The listing builds one solid part. Answer for the finished solid, in the listing's coordinates (mm). Face numbers are marked on the shaded views. A direction names the side the tool comes from. Coordinates: 2 decimals unless noted, no trailing zeros. Write each loop counter-clockwise with the first axis right and the second up, starting at its lowest first coordinate (ties: lowest second). Pieces come first, ordered by that corner, then holes.
(1) Which of the six approach directions +Z, -Z, +X, -X, +Y, -Y give full straight-line access (tool end or side, diameter ignored) to the marked faces 5, 6, 7 and 8?
(2) Straight lines are drawn through the part: line 1 (X direction, y = 89.4, z = 17.65); line 2 (Y direction, x = 0, z = 11.75); line 3 (Z direction, x = 12, y = 24). For each, find the intervals that lie inside material, in ascending order.
(3) The part is cut by section C-C on y = 30. Determine the outline of the cut face in (x, z), plus the area to 3 significant figures.
(4) The part is cut by section D-D on y = 13. Determine the outline of the cut face in (x, z).
(5) Given P1, Ø6, axis at x = 15.5, y = 37, coming from the -Z side; P2, Ø10, axis at y = 102.5, z = 6.5, coming from the +X side; P3, Ø4, axis at x = -10.5, y = 89.4, coming from the +Z side, each flat-ended and moving along its own axis, determine where each tip first touches the part or whether it passes through.
(6) The part is cut by section B-B on y = 103.9. Determine the outline of the cut face in (x, z).
(7) For a pull along X with two mould halves and no side action, classify the marked faces 1, 2, 3 and 4 as +X half, -X half, draft (parallel to the pull), parting line (faces both ways), or undercut.
(8) The part is cut by section A-A on z = 0. Determine the outline of the cut face in (x, y), plus the area to 3 significant figures.
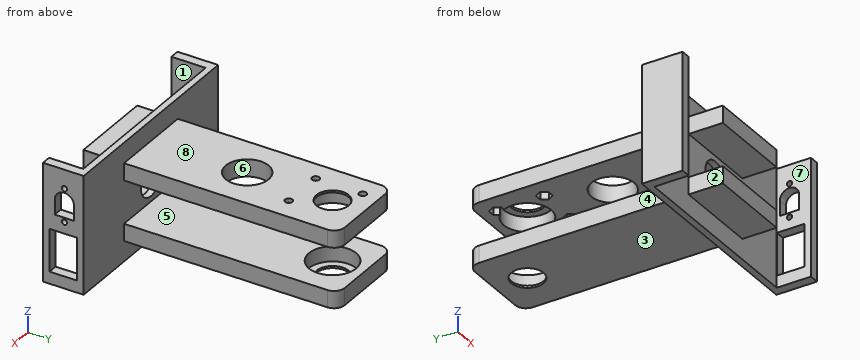
from build123d import *

# Parameters (mm, degrees)
SKETCH1_W            = 100
SKETCH1_H            = 55
BOSS_EXTRUDE1_DEPTH  = 19
SKETCH2_W            = 91
SKETCH2_H            = 91
CUT_EXTRUDE1_DEPTH   = 16
CUT_EXTRUDE3_REACH   = 102
SKETCH3_R            = 1.25
CUT_EXTRUDE13_REACH  = 102
SKETCH15_W           = 19.8
SKETCH15_H           = 12.9
BOSS_EXTRUDE2_START  = -19
SKETCH6_W            = 40
SKETCH6_H            = 8
BOSS_EXTRUDE2_DEPTH  = 119
SKETCH7_R            = 11.05
CUT_EXTRUDE5_DEPTH   = 7
SKETCH8_R            = 7.55
CUT_EXTRUDE6_DEPTH   = 1
FILLET1_R            = 5
FILLET1_OF_MIRROR2_R = 5
CUT_EXTRUDE7_REACH   = 21
SKETCH9_R            = 7.5
CUT_EXTRUDE10_REACH  = 47.5
SKETCH12_R           = 10
CUT_EXTRUDE11_REACH  = 47.5
SKETCH13_R           = 1.75
CUT_EXTRUDE12_DEPTH  = 6


with BuildPart() as part:
    # Sketch1 → Boss-Extrude1 (new body)
    with BuildSketch(Plane(origin=(0, 0, 0), x_dir=(1, 0, 0), z_dir=(0, 1, 0))):
        Rectangle(SKETCH1_W, SKETCH1_H)
    extrude(amount=BOSS_EXTRUDE1_DEPTH)

    # Sketch2 → Cut-Extrude1 (cut)
    with BuildSketch(Plane.XZ):
        Rectangle(SKETCH2_W, SKETCH2_H)
    extrude(amount=-CUT_EXTRUDE1_DEPTH, mode=Mode.SUBTRACT)

    # Sketch3 → Cut-Extrude3 (cut, up to next)
    with BuildSketch(Plane(origin=(50, 0, 0), x_dir=(0, 0, -1), z_dir=(1, 0, 0)), mode=Mode.PRIVATE) as cut_extrude3_sk1:
        with Locations((-18.75, 10)):
            Circle(SKETCH3_R)
    cut_extrude3_tool1 = extrude(cut_extrude3_sk1.sketch, amount=-CUT_EXTRUDE3_REACH, mode=Mode.PRIVATE) & part.part
    add(cut_extrude3_tool1.solids().sort_by_distance((50, 10, 18.75))[0], mode=Mode.SUBTRACT)
    # Sketch3 → Cut-Extrude3 (cut, up to next)
    with BuildSketch(Plane(origin=(50, 0, 0), x_dir=(0, 0, -1), z_dir=(1, 0, 0)), mode=Mode.PRIVATE) as cut_extrude3_sk2:
        with Locations((-3.25, 10)):
            Circle(SKETCH3_R)
    cut_extrude3_tool2 = extrude(cut_extrude3_sk2.sketch, amount=-CUT_EXTRUDE3_REACH, mode=Mode.PRIVATE) & part.part
    add(cut_extrude3_tool2.solids().sort_by_distance((50, 10, 3.25))[0], mode=Mode.SUBTRACT)
    # Sketch3 → Cut-Extrude3 (cut, up to next)
    with BuildSketch(Plane(origin=(50, 0, 0), x_dir=(0, 0, -1), z_dir=(1, 0, 0)), mode=Mode.PRIVATE) as cut_extrude3_sk3:
        with BuildLine():
            Line((-5.272727273, 5.5), (-5.272727273, 14.5))
            Line((-5.272727273, 14.5), (-12.278409091, 14.5))
            ThreePointArc((-12.278409091, 14.5), (-16.778409091, 10), (-12.278409091, 5.5))
            Line((-12.278409091, 5.5), (-5.272727273, 5.5))
        make_face()
    cut_extrude3_tool3 = extrude(cut_extrude3_sk3.sketch, amount=-CUT_EXTRUDE3_REACH, mode=Mode.PRIVATE) & part.part
    add(cut_extrude3_tool3.solids().sort_by_distance((50, 10, 10.590569))[0], mode=Mode.SUBTRACT)

    # Sketch15 → Cut-Extrude13 (cut, up to next)
    with BuildSketch(Plane(origin=(50, 0, 0), x_dir=(0, 0, -1), z_dir=(1, 0, 0)), mode=Mode.PRIVATE) as cut_extrude13_sk1:
        with Locations((12, 9.5)):
            Rectangle(SKETCH15_W, SKETCH15_H)
    cut_extrude13_tool1 = extrude(cut_extrude13_sk1.sketch, amount=-CUT_EXTRUDE13_REACH, mode=Mode.PRIVATE) & part.part
    add(cut_extrude13_tool1.solids().sort_by_distance((50, 9.5, -12))[0], mode=Mode.SUBTRACT)

    # Sketch6 → Boss-Extrude2 (add)
    with BuildSketch(Plane(origin=(0, 19, 0), x_dir=(1, 0, 0), z_dir=(0, 1, 0)).offset(BOSS_EXTRUDE2_START)):
        with Locations((0, -14)):
            Rectangle(SKETCH6_W, SKETCH6_H)
    boss_extrude2 = extrude(amount=BOSS_EXTRUDE2_DEPTH)

    # Sketch7 → Cut-Extrude5 (cut)
    with BuildSketch(Plane(origin=(0, 0, 10), x_dir=(-1, 0, 0), z_dir=(0, 0, -1))):
        with Locations((0, 103.9)):
            Circle(SKETCH7_R)
    cut_extrude5 = extrude(amount=-CUT_EXTRUDE5_DEPTH, mode=Mode.SUBTRACT)

    # Sketch8 → Cut-Extrude6 (cut)
    with BuildSketch(Plane.XY.offset(18)):
        with Locations((0, 103.9)):
            Circle(SKETCH8_R)
    cut_extrude6 = extrude(amount=-CUT_EXTRUDE6_DEPTH, mode=Mode.SUBTRACT)

    # Fillet1
    fillet1_edges = [part.edges().sort_by_distance(p)[0] for p in [
        (-20, 119, 14),
        (20, 119, 14),
    ]]
    fillet(fillet1_edges, radius=FILLET1_R)

    # Mirror2: Boss-Extrude2, Cut-Extrude5, Cut-Extrude6 across plane
    add(boss_extrude2.mirror(Plane.XY))
    add(cut_extrude5.mirror(Plane.XY), mode=Mode.SUBTRACT)
    add(cut_extrude6.mirror(Plane.XY), mode=Mode.SUBTRACT)

    # Fillet1 of Mirror2
    fillet1_of_mirror2_edges = [part.edges().sort_by_distance(p)[0] for p in [
        (-20, 119, -14),
        (20, 119, -14),
    ]]
    fillet(fillet1_of_mirror2_edges, radius=FILLET1_OF_MIRROR2_R)

    # Sketch9 → Cut-Extrude7 (cut, up to next)
    with BuildSketch(Plane(origin=(0, 19, 0), x_dir=(1, 0, 0), z_dir=(0, 1, 0)), mode=Mode.PRIVATE) as cut_extrude7_sk1:
        Circle(SKETCH9_R)
    cut_extrude7_tool1 = extrude(cut_extrude7_sk1.sketch, amount=-CUT_EXTRUDE7_REACH, mode=Mode.PRIVATE) & part.part
    add(cut_extrude7_tool1.solids().sort_by_distance((0, 19, 0))[0], mode=Mode.SUBTRACT)

    # Sketch12 → Cut-Extrude10 (cut, up to next)
    with BuildSketch(Plane.XY.offset(18), mode=Mode.PRIVATE) as cut_extrude10_sk1:
        with Locations((0, 64)):
            Circle(SKETCH12_R)
    cut_extrude10_tool1 = extrude(cut_extrude10_sk1.sketch, amount=-CUT_EXTRUDE10_REACH, mode=Mode.PRIVATE) & part.part
    add(cut_extrude10_tool1.solids().sort_by_distance((0, 64, 18))[0], mode=Mode.SUBTRACT)

    # Sketch13 → Cut-Extrude11 (cut, up to next)
    with BuildSketch(Plane.XY.offset(18), mode=Mode.PRIVATE) as cut_extrude11_sk1:
        with Locations((-10.5, 89.4)):
            Circle(SKETCH13_R)
    cut_extrude11_tool1 = extrude(cut_extrude11_sk1.sketch, amount=-CUT_EXTRUDE11_REACH, mode=Mode.PRIVATE) & part.part
    add(cut_extrude11_tool1.solids().sort_by_distance((-10.5, 89.4, 18))[0], mode=Mode.SUBTRACT)
    # Sketch13 → Cut-Extrude11 (cut, up to next)
    with BuildSketch(Plane.XY.offset(18), mode=Mode.PRIVATE) as cut_extrude11_sk2:
        with Locations((-10.5, 111.4)):
            Circle(SKETCH13_R)
    cut_extrude11_tool2 = extrude(cut_extrude11_sk2.sketch, amount=-CUT_EXTRUDE11_REACH, mode=Mode.PRIVATE) & part.part
    add(cut_extrude11_tool2.solids().sort_by_distance((-10.5, 111.4, 18))[0], mode=Mode.SUBTRACT)
    # Sketch13 → Cut-Extrude11 (cut, up to next)
    with BuildSketch(Plane.XY.offset(18), mode=Mode.PRIVATE) as cut_extrude11_sk3:
        with Locations((9.5, 89.4)):
            Circle(SKETCH13_R)
    cut_extrude11_tool3 = extrude(cut_extrude11_sk3.sketch, amount=-CUT_EXTRUDE11_REACH, mode=Mode.PRIVATE) & part.part
    add(cut_extrude11_tool3.solids().sort_by_distance((9.5, 89.4, 18))[0], mode=Mode.SUBTRACT)

    # Sketch14 → Cut-Extrude12 (cut)
    with BuildSketch(Plane(origin=(0, 0, 10), x_dir=(-1, 0, 0), z_dir=(0, 0, -1))):
        Polygon((-11.174315781, 92.3), (-7.825684219, 92.3), (-6.151368439, 89.4), (-7.825684219, 86.5), (-11.174315781, 86.5), (-12.848631561, 89.4), align=None)
        Polygon((13.848631561, 89.4), (12.174315781, 92.3), (8.825684219, 92.3), (7.151368439, 89.4), (8.825684219, 86.5), (12.174315781, 86.5), align=None)
        Polygon((7.151368439, 111.4), (8.825684219, 114.3), (12.174315781, 114.3), (13.848631561, 111.4), (12.174315781, 108.5), (8.825684219, 108.5), align=None)
    extrude(amount=-CUT_EXTRUDE12_DEPTH, mode=Mode.SUBTRACT)


solid = part.part
Model answer:
1. face 5: +X, -X, +Y
1. face 6: +Z
1. face 7: +Z, -Z, -Y
1. face 8: +Z, +X, -X, +Y
2. line 1: x = -20 to -12.25, -8.75 to 7.75, 11.25 to 20
2. line 2: y = 0 to 54, 74 to 92.85, 114.95 to 119
2. line 3: z = -18 to -10, 10 to 18
3. outline: (-20, -18) - (20, -18) - (20, -10) - (-20, -10) - close; (-20, 10) - (20, 10) - (20, 18) - (-20, 18) - close
3. area: 640 mm2
4. outline: (-50, -27.5) - (-45.5, -27.5) - (-45.5, 27.5) - (-50, 27.5) - close; (-20, -18) - (20, -18) - (20, -10) - (-20, -10) - close; (-20, 10) - (20, 10) - (20, 18) - (-20, 18) - close; (45.5, -27.5) - (50, -27.5) - (50, -21.9) - (45.5, -21.9) - close; (45.5, -2.1) - (50, -2.1) - (50, 5.27) - (45.5, 5.27) - close; (45.5, 15.63) - (50, 15.63) - (50, 27.5) - (45.5, 27.5) - close
5. P1: stops at z = -18
5. P2: stops at x = 20
5. P3: stops at z = 18
6. outline: (-20, -18) - (-7.55, -18) - (-7.55, -17) - (-11.05, -17) - (-11.05, -10) - (-20, -10) - close; (-20, 10) - (-11.05, 10) - (-11.05, 17) - (-7.55, 17) - (-7.55, 18) - (-20, 18) - close; (7.55, -18) - (20, -18) - (20, -10) - (11.05, -10) - (11.05, -17) - (7.55, -17) - close; (7.55, 17) - (11.05, 17) - (11.05, 10) - (20, 10) - (20, 18) - (7.55, 18) - close
7. face 1: undercut
7. face 2: undercut
7. face 3: draft
7. face 4: -X half
8. outline: (-50, 0) - (-45.5, 0) - (-45.5, 16) - (-7.5, 16) - (-7.5, 19) - (-50, 19) - close; (7.5, 16) - (45.5, 16) - (45.5, 0) - (50, 0) - (50, 19) - (7.5, 19) - close
8. area: 399 mm2
